Build history of the part. All positions in model axes, mm. A direction names the side the tool comes from. Give positions to 0.01 mm unless a question says otherwise; leave off trailing zeros. Order: outer loops, then holes, each group sorted by start corner. A loop starts at its lowest first (then second) coordinate and runs counter-clockwise, first axis right, second up. Notation, with made-up numbers: M -38,67.25 L -8,67.25 A7 cw -8,72.25 Z; hole C -17.5,25 d2. An arc over 180 degrees is marked long. One line per item, written item: value. Start each with the question number.
Autodesk Inventor part; units mm, degrees
ref_plane "YZ Plane" through (0, 0, 0) normal (1, 0, 0) x (0, 1, 0)
ref_plane "XZ Plane" through (0, 0, 0) normal (0, 1, 0) x (-1, 0, 0)
ref_plane "XY Plane" through (0, 0, 0) normal (0, 0, 1) x (1, 0, 0)
sketch "Sketch1" plane through (0, 0, 0) normal (0, 0, 1) x (1, 0, 0)
  line L0 (0, 0) -> (304.8, 0)
  line L1 (304.8, 0) -> (304.8, 133.35)
  line L2 (304.8, 133.35) -> (0, 133.35)
  line L3 (0, 133.35) -> (0, 0)
  dimension "d0" = 304.8
  dimension "d1" = 133.35
extrude "Extrusion1" add sketch "Sketch1" along normal blind 19.05
sketch "Sketch2" plane through (0, 0, 19.05) normal (0, 0, 1) x (1, 0, 0)
  line L0 (304.8, 133.35) -> (0, 133.35)
  line L1 (0, 133.35) -> (0, 0)
  line L2 (82.55, 133.35) -> (222.25, 133.35)
  line L3 (222.25, 133.35) -> (222.25, 114.3)
  line L4 (222.25, 114.3) -> (82.55, 114.3)
  line L5 (82.55, 114.3) -> (82.55, 133.35)
  dimension "d4" = 139.7
  dimension "d5" = 19.05
  dimension "d6" = 82.55
extrude "Extrusion2" add sketch "Sketch2" along normal blind 165.1
sketch "Sketch3" plane through (82.55, 114.3, 19.05) normal (0, -1, 0) x (1, 0, 0)
  line L0 (0, 165.1) -> (139.7, 165.1)
  circle A0 centre (69.85, 152.4) radius 9.525
  point P0 (-82.55, -19.05)
  dimension "d9" = 19.05
  dimension "d10" = 12.7
extrude "Extrusion3" cut sketch "Sketch3" against normal blind 165.1
properties part number "Puller1"
1) Slice it at C-C (y = 36.5). List the corners of the cut face in (x, z).
2) Slice it at A-A (z = 171.45). List the corners of the cut face in (x, y) (3 decimals).
3) Drill centre lines: line 1 (X direction, y = 125, z = 171); line 2 (Z direction, x = 152, y = 124); line 3 (Y direction, x = 159, z = 120). Where is each one in solid material? Low to high.
4) Drop flat-ended pins along their axis: P1, Ø9.5, axis at y = 128.5, z = 134.5, coming from the -X side; P2, Ø12, axis at x = 185.5, y = 32.5, coming from the +Z side; P3, Ø10, axis at x = 171.5, z = 104, coming from the -Y side. Give the stop position or say it passes through.
5) Tool access for faces 1 (the flat face through (82.55, 124, 100)), 2 (the flat face through (222.25, 124, 100)), 3 (the flat face through (153, 114.3, 100)): list every direction of +Z, -Z, +X, -X, +Y, -Y with a clear straight run to the whole face (end or side of a thin tool).
6) Slice it at D-D (z = 93). List the corners of the cut face in (x, y), plus the area to 3 significant figures.
7) Slice it at B-B (x = 152.4). List the corners of the cut face in (y, z) (3 decimals), plus the area to 3 significant figures.
Results list:
1. outline: M 0,0 L 304.8,0 L 304.8,19.05 L 0,19.05 Z
2. outline: M 82.55,114.3 L 142.875,114.3 L 142.875,133.35 L 82.55,133.35 Z; M 161.925,114.3 L 222.25,114.3 L 222.25,133.35 L 161.925,133.35 Z
3. line 1: x = 82.55 to 142.89, 161.91 to 222.25
3. line 2: z = 0 to 161.93, 180.97 to 184.15
3. line 3: y = 114.3 to 133.35
4. P1: stops at x = 82.55
4. P2: stops at z = 19.05
4. P3: stops at y = 114.3
5. face 1: +Z, -X, +Y, -Y
5. face 2: +Z, +X, +Y, -Y
5. face 3: +Z, +X, -X, -Y
6. outline: M 82.55,114.3 L 222.25,114.3 L 222.25,133.35 L 82.55,133.35 Z
6. area: 2,660 mm²
7. outline: M 0,0 L 133.35,0 L 133.35,161.925 L 114.3,161.925 L 114.3,19.05 L 0,19.05 Z; M 114.3,180.975 L 133.35,180.975 L 133.35,184.15 L 114.3,184.15 Z
7. area: 5,320 mm²
